from build123d import *

# Parameters (mm, degrees)
CROQUIS1_W              = 40
CROQUIS1_H              = 70
SALIENTE_EXTRUIR1_DEPTH = 1
REDONDEO1_R             = 10
CORTAR_EXTRUIR1_REACH   = 50.527
CROQUIS2_R              = 0.75
CROQUIS5_W              = 32.8
CROQUIS5_H              = 13
SALIENTE_EXTRUIR2_DEPTH = 12
VACIADO1_START          = -15.316182085
VACIADO1_OUTLINE_W      = 11
VACIADO1_OUTLINE_H      = 12
VACIADO1_DEPTH          = 30.8
CORTAR_EXTRUIR4_REACH   = 51.979
CROQUIS6_W              = 1
CROQUIS6_H              = 4
CROQUIS7_W              = 32.3
CROQUIS7_H              = 12.5
CORTAR_EXTRUIR5_DEPTH   = 1
CROQUIS8_W              = 4.2
CROQUIS8_H              = 4
CORTAR_EXTRUIR6_DEPTH   = 0.6
REDONDEO2_R             = 1
REDONDEO3_R             = 0.3
CROQUIS9_W              = 4.2
CROQUIS9_H              = 1.65
CORTAR_EXTRUIR7_DEPTH   = 1.2
CROQUIS10_W             = 2
CROQUIS10_H             = 0.5
CORTAR_EXTRUIR8_DEPTH   = 1.5
CROQUIS11_R             = 1.25
CORTAR_EXTRUIR9_DEPTH   = 0.6
SALIENTE_EXTRUIR3_REACH = 51.979
CROQUIS12_W             = 0.5
CROQUIS12_H             = 2


# Read off the part's stored shape, not the designer's step: Vaciado1
with BuildPart() as part:
    # Croquis1 → Saliente-Extruir1 (new body)
    with BuildSketch(Plane.XY):
        with Locations((0.083817915, -9.164456233)):
            Rectangle(CROQUIS1_W, CROQUIS1_H)
    extrude(amount=SALIENTE_EXTRUIR1_DEPTH)

    # Redondeo1
    redondeo1_edges = [part.edges().sort_by_distance(p)[0] for p in [
        (-19.916182085, 25.835543767, 0.5),
        (20.083817915, 25.835543767, 0.5),
    ]]
    fillet(redondeo1_edges, radius=REDONDEO1_R)

    # Croquis2 → Cortar-Extruir1 (cut, up to next)
    with BuildSketch(Plane(origin=(0, 0, 0), x_dir=(-1, 0, 0), z_dir=(0, 0, -1)), mode=Mode.PRIVATE) as cortar_extruir1_sk1:
        with Locations((-5.583817915, 24.085543767)):
            Circle(CROQUIS2_R)
    cortar_extruir1_tool1 = extrude(cortar_extruir1_sk1.sketch, amount=-CORTAR_EXTRUIR1_REACH, mode=Mode.PRIVATE) & part.part
    # Croquis2 → Cortar-Extruir1 (cut, up to next)
    with BuildSketch(Plane(origin=(0, 0, 0), x_dir=(-1, 0, 0), z_dir=(0, 0, -1)), mode=Mode.PRIVATE) as cortar_extruir1_sk2:
        with Locations((5.416182085, 24.085543767)):
            Circle(CROQUIS2_R)
    cortar_extruir1_tool2 = extrude(cortar_extruir1_sk2.sketch, amount=-CORTAR_EXTRUIR1_REACH, mode=Mode.PRIVATE) & part.part
    # Croquis2 → Cortar-Extruir1 (cut, up to next)
    with BuildSketch(Plane(origin=(0, 0, 0), x_dir=(-1, 0, 0), z_dir=(0, 0, -1)), mode=Mode.PRIVATE) as cortar_extruir1_sk3:
        with Locations((-18.183817915, -42.414456233)):
            Circle(CROQUIS2_R)
    cortar_extruir1_tool3 = extrude(cortar_extruir1_sk3.sketch, amount=-CORTAR_EXTRUIR1_REACH, mode=Mode.PRIVATE) & part.part
    # Croquis2 → Cortar-Extruir1 (cut, up to next)
    with BuildSketch(Plane(origin=(0, 0, 0), x_dir=(-1, 0, 0), z_dir=(0, 0, -1)), mode=Mode.PRIVATE) as cortar_extruir1_sk4:
        with Locations((-0.083817915, -42.414456233)):
            Circle(CROQUIS2_R)
    cortar_extruir1_tool4 = extrude(cortar_extruir1_sk4.sketch, amount=-CORTAR_EXTRUIR1_REACH, mode=Mode.PRIVATE) & part.part
    # Croquis2 → Cortar-Extruir1 (cut, up to next)
    with BuildSketch(Plane(origin=(0, 0, 0), x_dir=(-1, 0, 0), z_dir=(0, 0, -1)), mode=Mode.PRIVATE) as cortar_extruir1_sk5:
        with Locations((18.016182085, -42.414456233)):
            Circle(CROQUIS2_R)
    cortar_extruir1_tool5 = extrude(cortar_extruir1_sk5.sketch, amount=-CORTAR_EXTRUIR1_REACH, mode=Mode.PRIVATE) & part.part
    # Croquis2 → Cortar-Extruir1 (cut, up to next)
    with BuildSketch(Plane(origin=(0, 0, 0), x_dir=(-1, 0, 0), z_dir=(0, 0, -1)), mode=Mode.PRIVATE) as cortar_extruir1_sk6:
        with Locations((-18.333817915, 12.585543767)):
            Circle(CROQUIS2_R)
    cortar_extruir1_tool6 = extrude(cortar_extruir1_sk6.sketch, amount=-CORTAR_EXTRUIR1_REACH, mode=Mode.PRIVATE) & part.part
    # Croquis2 → Cortar-Extruir1 (cut, up to next)
    with BuildSketch(Plane(origin=(0, 0, 0), x_dir=(-1, 0, 0), z_dir=(0, 0, -1)), mode=Mode.PRIVATE) as cortar_extruir1_sk7:
        with Locations((-18.333817915, -22.414456233)):
            Circle(CROQUIS2_R)
    cortar_extruir1_tool7 = extrude(cortar_extruir1_sk7.sketch, amount=-CORTAR_EXTRUIR1_REACH, mode=Mode.PRIVATE) & part.part
    # Croquis2 → Cortar-Extruir1 (cut, up to next)
    with BuildSketch(Plane(origin=(0, 0, 0), x_dir=(-1, 0, 0), z_dir=(0, 0, -1)), mode=Mode.PRIVATE) as cortar_extruir1_sk8:
        with Locations((18.166182085, 12.585543767)):
            Circle(CROQUIS2_R)
    cortar_extruir1_tool8 = extrude(cortar_extruir1_sk8.sketch, amount=-CORTAR_EXTRUIR1_REACH, mode=Mode.PRIVATE) & part.part
    # Croquis2 → Cortar-Extruir1 (cut, up to next)
    with BuildSketch(Plane(origin=(0, 0, 0), x_dir=(-1, 0, 0), z_dir=(0, 0, -1)), mode=Mode.PRIVATE) as cortar_extruir1_sk9:
        with Locations((18.166182085, -22.414456233)):
            Circle(CROQUIS2_R)
    cortar_extruir1_tool9 = extrude(cortar_extruir1_sk9.sketch, amount=-CORTAR_EXTRUIR1_REACH, mode=Mode.PRIVATE) & part.part
    add(cortar_extruir1_tool1.solids().sort_by_distance((5.583818, 24.085544, 0))[0], mode=Mode.SUBTRACT)
    add(cortar_extruir1_tool2.solids().sort_by_distance((-5.416182, 24.085544, 0))[0], mode=Mode.SUBTRACT)
    add(cortar_extruir1_tool3.solids().sort_by_distance((18.183818, -42.414456, 0))[0], mode=Mode.SUBTRACT)
    add(cortar_extruir1_tool4.solids().sort_by_distance((0.083818, -42.414456, 0))[0], mode=Mode.SUBTRACT)
    add(cortar_extruir1_tool5.solids().sort_by_distance((-18.016182, -42.414456, 0))[0], mode=Mode.SUBTRACT)
    add(cortar_extruir1_tool6.solids().sort_by_distance((18.333818, 12.585544, 0))[0], mode=Mode.SUBTRACT)
    add(cortar_extruir1_tool7.solids().sort_by_distance((18.333818, -22.414456, 0))[0], mode=Mode.SUBTRACT)
    add(cortar_extruir1_tool8.solids().sort_by_distance((-18.166182, 12.585544, 0))[0], mode=Mode.SUBTRACT)
    add(cortar_extruir1_tool9.solids().sort_by_distance((-18.166182, -22.414456, 0))[0], mode=Mode.SUBTRACT)

    # Croquis5 → Saliente-Extruir2 (add)
    with BuildSketch(Plane.XY.offset(1)):
        with Locations((0.083817915, 7.335543767)):
            Rectangle(CROQUIS5_W, CROQUIS5_H)
    extrude(amount=SALIENTE_EXTRUIR2_DEPTH)

    # Vaciado1 outline → Vaciado1 (cut)
    with BuildSketch(Plane.YZ.offset(VACIADO1_START)):
        with Locations((7.335543767, 6)):
            Rectangle(VACIADO1_OUTLINE_W, VACIADO1_OUTLINE_H)
    extrude(amount=VACIADO1_DEPTH, mode=Mode.SUBTRACT)

    # Croquis6 → Cortar-Extruir4 (cut, up to next)
    with BuildSketch(Plane(origin=(0, 0, 12), x_dir=(-1, 0, 0), z_dir=(0, 0, -1)), mode=Mode.PRIVATE) as cortar_extruir4_sk1:
        with Locations((-14.983817915, 7.335543767)):
            Rectangle(CROQUIS6_W, CROQUIS6_H)
    cortar_extruir4_tool1 = extrude(cortar_extruir4_sk1.sketch, amount=-CORTAR_EXTRUIR4_REACH, mode=Mode.PRIVATE) & part.part
    # Croquis6 → Cortar-Extruir4 (cut, up to next)
    with BuildSketch(Plane(origin=(0, 0, 12), x_dir=(-1, 0, 0), z_dir=(0, 0, -1)), mode=Mode.PRIVATE) as cortar_extruir4_sk2:
        with Locations((14.816182085, 7.335543767)):
            Rectangle(CROQUIS6_W, CROQUIS6_H)
    cortar_extruir4_tool2 = extrude(cortar_extruir4_sk2.sketch, amount=-CORTAR_EXTRUIR4_REACH, mode=Mode.PRIVATE) & part.part
    add(cortar_extruir4_tool1.solids().sort_by_distance((14.983818, 7.335544, 12))[0], mode=Mode.SUBTRACT)
    add(cortar_extruir4_tool2.solids().sort_by_distance((-14.816182, 7.335544, 12))[0], mode=Mode.SUBTRACT)

    # Croquis7 → Cortar-Extruir5 (cut)
    with BuildSketch(Plane(origin=(0, 0, 0), x_dir=(-1, 0, 0), z_dir=(0, 0, -1))):
        with Locations((-0.083817915, 7.335543767)):
            Rectangle(CROQUIS7_W, CROQUIS7_H)
    extrude(amount=-CORTAR_EXTRUIR5_DEPTH, mode=Mode.SUBTRACT)

    # Croquis8 → Cortar-Extruir6 (cut)
    with BuildSketch(Plane(origin=(0, 0, 0), x_dir=(-1, 0, 0), z_dir=(0, 0, -1))):
        with Locations((-0.083817915, 15.585543767)):
            Rectangle(CROQUIS8_W, CROQUIS8_H)
    extrude(amount=-CORTAR_EXTRUIR6_DEPTH, mode=Mode.SUBTRACT)

    # Redondeo2
    redondeo2_edges = [part.edges().sort_by_distance(p)[0] for p in [
        (2.183817915, 17.585543767, 0.3),
        (-2.016182085, 17.585543767, 0.3),
    ]]
    fillet(redondeo2_edges, radius=REDONDEO2_R)

    # Redondeo3
    redondeo3_edges = [part.edges().sort_by_distance(p)[0] for p in [
        (-2.016182085, 15.085543767, 0),
        (0.083817915, 17.585543767, 0),
        (2.183817915, 15.085543767, 0),
        (-1.723288867, 17.292650548, 0),
        (1.890924696, 17.292650548, 0),
    ]]
    fillet(redondeo3_edges, radius=REDONDEO3_R)

    # Croquis9 → Cortar-Extruir7 (cut)
    with BuildSketch(Plane(origin=(0, 0, 0.6), x_dir=(-1, 0, 0), z_dir=(0, 0, -1))):
        with Locations((-0.083817915, 14.310543767)):
            Rectangle(CROQUIS9_W, CROQUIS9_H)
    extrude(amount=-CORTAR_EXTRUIR7_DEPTH, mode=Mode.SUBTRACT)

    # Croquis10 → Cortar-Extruir8 (cut)
    with BuildSketch(Plane(origin=(0, 1.085543767, 0), x_dir=(1, 0, 0), z_dir=(0, 1, 0))):
        with Locations((-13.066182085, -0.75)):
            Rectangle(CROQUIS10_W, CROQUIS10_H)
        with Locations((13.233817915, -0.75)):
            Rectangle(CROQUIS10_W, CROQUIS10_H)
    extrude(amount=-CORTAR_EXTRUIR8_DEPTH, mode=Mode.SUBTRACT)

    # Croquis11 → Cortar-Extruir9 (cut)
    with BuildSketch(Plane(origin=(0, 0, 0), x_dir=(-1, 0, 0), z_dir=(0, 0, -1))):
        with Locations((-5.583817915, 24.085543767)):
            Circle(CROQUIS11_R)
        with Locations((5.416182085, 24.085543767)):
            Circle(CROQUIS11_R)
        with Locations((18.166182085, 12.585543767)):
            Circle(CROQUIS11_R)
        with Locations((-18.333817915, 12.585543767)):
            Circle(CROQUIS11_R)
        with Locations((-18.333817915, -22.414456233)):
            Circle(CROQUIS11_R)
        with Locations((18.166182085, -22.414456233)):
            Circle(CROQUIS11_R)
        with Locations((18.016182085, -42.414456233)):
            Circle(CROQUIS11_R)
        with Locations((-0.083817915, -42.414456233)):
            Circle(CROQUIS11_R)
        with Locations((-18.183817915, -42.414456233)):
            Circle(CROQUIS11_R)
    extrude(amount=-CORTAR_EXTRUIR9_DEPTH, mode=Mode.SUBTRACT)

    # Croquis12 → Saliente-Extruir3 (add, up to next)
    with BuildSketch(Plane(origin=(0, 0, 1), x_dir=(-1, 0, 0), z_dir=(0, 0, -1)), mode=Mode.PRIVATE) as saliente_extruir3_sk1:
        with Locations((-14.733817915, 11.835543767)):
            Rectangle(CROQUIS12_W, CROQUIS12_H)
    saliente_extruir3_tool1 = extrude(saliente_extruir3_sk1.sketch, amount=-SALIENTE_EXTRUIR3_REACH, mode=Mode.PRIVATE) - part.part
    # Croquis12 → Saliente-Extruir3 (add, up to next)
    with BuildSketch(Plane(origin=(0, 0, 1), x_dir=(-1, 0, 0), z_dir=(0, 0, -1)), mode=Mode.PRIVATE) as saliente_extruir3_sk2:
        with Locations((-14.733817915, 2.835543767)):
            Rectangle(CROQUIS12_W, CROQUIS12_H)
    saliente_extruir3_tool2 = extrude(saliente_extruir3_sk2.sketch, amount=-SALIENTE_EXTRUIR3_REACH, mode=Mode.PRIVATE) - part.part
    # Croquis12 → Saliente-Extruir3 (add, up to next)
    with BuildSketch(Plane(origin=(0, 0, 1), x_dir=(-1, 0, 0), z_dir=(0, 0, -1)), mode=Mode.PRIVATE) as saliente_extruir3_sk3:
        with Locations((14.566182085, 11.835543767)):
            Rectangle(CROQUIS12_W, CROQUIS12_H)
    saliente_extruir3_tool3 = extrude(saliente_extruir3_sk3.sketch, amount=-SALIENTE_EXTRUIR3_REACH, mode=Mode.PRIVATE) - part.part
    # Croquis12 → Saliente-Extruir3 (add, up to next)
    with BuildSketch(Plane(origin=(0, 0, 1), x_dir=(-1, 0, 0), z_dir=(0, 0, -1)), mode=Mode.PRIVATE) as saliente_extruir3_sk4:
        with Locations((14.566182085, 2.835543767)):
            Rectangle(CROQUIS12_W, CROQUIS12_H)
    saliente_extruir3_tool4 = extrude(saliente_extruir3_sk4.sketch, amount=-SALIENTE_EXTRUIR3_REACH, mode=Mode.PRIVATE) - part.part
    add(saliente_extruir3_tool1.solids().sort_by_distance((14.733818, 11.835544, 1))[0])
    add(saliente_extruir3_tool2.solids().sort_by_distance((14.733818, 2.835544, 1))[0])
    add(saliente_extruir3_tool3.solids().sort_by_distance((-14.566182, 11.835544, 1))[0])
    add(saliente_extruir3_tool4.solids().sort_by_distance((-14.566182, 2.835544, 1))[0])


solid = part.part
Input: part model. Units: mm. Frame: model coordinates. A direction names the side the tool comes from. Coordinates: 2 decimals unless noted, no trailing zeros. Order: outer loops, then holes, each group sorted by start corner. A loop starts at its lowest first (then second) coordinate and runs counter-clockwise, first axis right, second up. Notation, with made-up numbers: M 33,20.5 L 48,20.5 A12 cw 48,41.5 Z; hole C 24,28 d6. An arc over 180 degrees is marked long. Write item = value, one per line. Start each with the question number.
(1) Reachability of faces 1 (the flat face through (19, -43, 0.6)), 2 (the flat face through (13, 0, 0.5)), 3 (the cylindrical face through (5.68, 24.83, 0.8)) from +Z, -Z, +X, -X, +Y, -Y: full face, straight path, thin tool, end or side. Return the list, or none.
(2) Section A-A on x = -3.5. Output: boundary loops of the cut face in (y, z), and give its area (3 significant figures).
(3) Section C-C on x = 5.5. Output: boundary loops of the cut face in (y, z), and give its area (3 significant figures).
(4) Section B-B on z = 7.5. Output: boundary loops of the cut face in (x, y), and give its area (3 significant figures).
(5) Pull-direction query (X, two-part tool) for faces 4 (the flat face through (0, -9, 1)), 5 (the cylindrical face through (19.583, 12.641, 0.296)), 6 (the flat face through (-16.316, 7, 7)); classes: released by +X, released by -X, zero draft, split by the parting line, or undercut.
(6) Section D-D on y = -29.5. Output: boundary loops of the cut face in (x, z).
(7) Line query: line 1 along Y through (x, z) = (11.5, 8.75); line 2 along X through (y, z) = (8.5, 2.5); line 3 along Z through (x, y) = (3, -32). Output: solid intervals per line, ascending. Write a range as [from, to].
(8) First-contact query: P1, Ø0.8, axis at x = 15, z = 12.5, coming from the +Y side; P2, Ø3, axis at x = 2.5, z = 7.5, coming from the -Y side; P3, Ø3, axis at x = -11.5, y = -32.5, coming from the +Z side. Flat tips, straight axial feed; report the tip coordinate or a pass-through.
Result set:
q1.face_1 = -Z
q1.face_2 = none
q1.face_3 = +Z, -Z
q2.outline = M -44.16,0 L 1.09,0 L 1.09,1 L 1.84,1 L 1.84,12 L 12.84,12 L 12.84,1 L 13.59,1 L 13.59,0 L 25.84,0 L 25.84,1 L 13.84,1 L 13.84,13 L 0.84,13 L 0.84,1 L -44.16,1 Z
q2.area = 92.5 mm²
q3.outline = M -44.16,0 L 1.09,0 L 1.09,1 L 1.84,1 L 1.84,12 L 12.84,12 L 12.84,1 L 13.59,1 L 13.59,0 L 22.84,0 L 22.84,0.6 L 23.34,0.6 L 23.34,1 L 13.84,1 L 13.84,13 L 0.84,13 L 0.84,1 L -44.16,1 Z; M 24.83,0.6 L 25.33,0.6 L 25.33,0 L 25.84,0 L 25.84,1 L 24.83,1 Z
q3.area = 90.4 mm²
q4.outline = M -16.32,0.84 L 16.48,0.84 L 16.48,13.84 L -16.32,13.84 Z; hole M -15.32,1.84 L -14.82,1.84 L -14.82,3.84 L -14.32,3.84 L -14.32,1.84 L 14.48,1.84 L 14.48,3.84 L 14.98,3.84 L 14.98,1.84 L 15.48,1.84 L 15.48,12.84 L 14.98,12.84 L 14.98,10.84 L 14.48,10.84 L 14.48,12.84 L -14.32,12.84 L -14.32,10.84 L -14.82,10.84 L -14.82,12.84 L -15.32,12.84 Z
q4.area = 91.6 mm²
q5.face_4 = zero draft
q5.face_5 = undercut
q5.face_6 = released by -X
q6.outline = M -19.92,0 L 20.08,0 L 20.08,1 L -19.92,1 Z
q7.line_1 = [0.84, 1.84], [12.84, 13.84]
q7.line_2 = [-16.32, -15.32], [15.48, 16.48]
q7.line_3 = [0, 1]
q8.P1 = 13.84
q8.P2 = 0.84
q8.P3 = 1
